from build123d import *

# Parameters (mm, degrees)
BASPROSKE_W        = 12
BASPROSKE_H        = 10.5
TOOTHCUT_DEPTH     = 20.091883092
TEETHCUTS_COUNT    = 12
TEETHCUTS_ANGLE    = 330
BORSKE_R           = 1.5
BORE_DEPTH         = 50.0000508
CUT_EXTRUDE1_DEPTH = 15


with BuildPart() as part:
    # BasProSke → Base-Revolve (revolve)
    with BuildSketch(Plane(origin=(0, 0, 0), x_dir=(1, 0, 0), z_dir=(0, 1, 0)), mode=Mode.PRIVATE) as base_revolve_sk:
        with Locations((6, 5.25)):
            Rectangle(BASPROSKE_W, BASPROSKE_H)
    revolve(base_revolve_sk.sketch.rotate(Axis((-10, 0, 0), (1, 0, 0)), 180), axis=Axis((-10, 0, 0), (1, 0, 0)))

    # TooCutSke → ToothCut (cut, through all)
    with BuildSketch(Plane(origin=(0, 0, 0), x_dir=(0, 0, -1), z_dir=(1, 0, 0))):
        with BuildLine():
            ThreePointArc((0.968931207, 7.05780053), (0, 7.124), (-0.968931207, 7.05780053))
            ThreePointArc((-0.968931207, 7.05780053), (-1.23511503, 8.836576748), (-2.328591557, 10.264585063))
            ThreePointArc((-2.328591557, 10.264585063), (0, 10.5254), (2.328591557, 10.264585063))
            ThreePointArc((2.328591557, 10.264585063), (1.23511503, 8.836576748), (0.968931207, 7.05780053))
        make_face()
    toothcut = extrude(amount=TOOTHCUT_DEPTH, mode=Mode.SUBTRACT)

    # TeethCuts: ToothCut ×12 about axis
    teethcuts_axis = Axis((-10, 0, 0), (1, 0, 0))
    for i in range(1, TEETHCUTS_COUNT):
        add(toothcut.rotate(teethcuts_axis, i * TEETHCUTS_ANGLE / (TEETHCUTS_COUNT - 1)), mode=Mode.SUBTRACT)

    # BorSke → Bore (cut, symmetric)
    with BuildSketch(Plane(origin=(0, 0, 0), x_dir=(0, 0, -1), z_dir=(1, 0, 0))):
        with Locations(Location((0, 0, 0), (0, 0, 180))):
            Circle(BORSKE_R)
    extrude(amount=BORE_DEPTH, both=True, mode=Mode.SUBTRACT)

    # Sketch1 → Cut-Extrude1 (cut)
    with BuildSketch(Plane(origin=(12, 0, 0), x_dir=(0, 0, -1), z_dir=(1, 0, 0))):
        with BuildLine():
            Line((1.540634556, -2.067724259), (1.540634556, 1.932275741))
            ThreePointArc((1.540634556, 1.932275741), (0.040634556, 2.432275741), (-1.459365444, 1.932275741))
            Line((-1.459365444, 1.932275741), (-1.459365444, -2.067724259))
            ThreePointArc((-1.459365444, -2.067724259), (0.040634556, -2.567724259), (1.540634556, -2.067724259))
        make_face()
    extrude(amount=-CUT_EXTRUDE1_DEPTH, mode=Mode.SUBTRACT)


solid = part.part
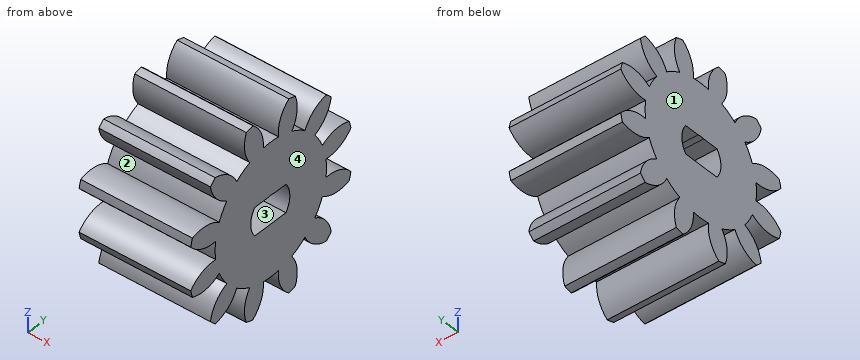
Geometry: final body of the model. Coordinates: model frame, mm. Face numbers are marked on the shaded views. A direction names the side the tool comes from. Coordinates: 2 decimals unless noted, no trailing zeros. Order: outer loops, then holes, each group sorted by start corner. A loop starts at its lowest first (then second) coordinate and runs counter-clockwise, first axis right, second up. Notation, with made-up numbers: M 68.5,64 L 72.5,64 A36 cw 72.5,100 Z; hole C 37.25,76 d6. An arc over 180 degrees is marked long. One line per question, with ' | ' between items. Start each with the question number.
Item 1: Set-up query: the marked faces 3 and 4. Return all of +Z, -Z, +X, -X, +Y, -Y with unobstructed straight access to the full face (end or side cutting, diameter ignored); none if empty.
Item 2: Cut plane D-D, the plane y = -4.75. Return the cut outline in (x, z), then the cut area to 3 significant figures.
Item 3: Cut plane B-B, the plane z = -9. Return the cut outline in (x, y).
Item 4: Ray query, probe 1 along Z at (x, y) = (7.25, -7.25); probe 2 along Z at (x, y) = (2.5, 0); probe 3 along Y at (x, z) = (10.25, 7). Return the intervals inside material, ascending. Write a range as [from, to].
Item 5: Cut plane C-C, the plane z = 6.25. Return the cut outline in (x, y), then the cut area to 3 significant figures.
Item 6: Pin query (flat end, axial travel): pin 1 Ø0.5 at (x, y) = (5.5, -1) entering from -Z; pin 2 Ø1.3 at (x, y) = (5, 1) entering from -Z; pin 3 Ø5 at (x, y) = (8, 7) entering from -Z. Return the tip coordinate at first contact, or that it passes through.
Item 7: Draft query along Y for the marked faces 1 and 2. Return one class per face: released by +Y, released by -Y, zero draft, split by the parting line, or undercut.
Item 8: Cut plane A-A, the plane y = 9.25. Return the cut outline in (x, z) (3 decimals).
A:
1) face 3: +X, -X | face 4: +Z, -Z, +X, +Y, -Y
2) outline: M 0,-6.29 L 12,-6.29 L 12,6.29 L 0,6.29 Z | area: 151 mm2
3) outline: M 0,-3.36 L 12,-3.36 L 12,-1.31 L 0,-1.31 Z; M 0,1.31 L 12,1.31 L 12,3.36 L 0,3.36 Z
4) probe 1: z = [-7.6, -5.81], [-3.07, -0.95], [0.95, 3.07], [5.81, 7.6] | probe 2: z = [-7.12, -1.54], [1.5, 7.12] | probe 3: y = [-7.7, -5.44], [-2.94, 2.94], [5.44, 7.7]
5) outline: M 0,-7.48 L 12,-7.48 L 12,-4.72 L 0,-4.72 Z; M 0,-3.42 L 12,-3.42 L 12,3.42 L 0,3.42 Z; M 0,4.72 L 12,4.72 L 12,7.48 L 0,7.48 Z | area: 148 mm2
6) pin 1: stops at z = -8.87 | pin 2: stops at z = -9.57 | pin 3: stops at z = -7.72
7) face 1: zero draft | face 2: undercut
8) outline: M 0,-3.335 L 12,-3.335 L 12,-1.443 L 0,-1.443 Z; M 0,1.443 L 12,1.443 L 12,3.335 L 0,3.335 Z
